Model file for the job. Use its own axes, mm. A direction names the side the tool comes from. Round coordinates to 2 decimals unless told otherwise and drop trailing zeros. Order: outer loops, then holes, each group sorted by start corner. A loop starts at its lowest first (then second) coordinate and runs counter-clockwise, first axis right, second up. Notation, with made-up numbers: (29, 55) -> (60, 55) arc R14 ccw to (60, 76) -> close; hole circle Ø8 at (-14, -20.75). An arc over 180 degrees is marked (long way). Put each result on its own line as item: value. Start each with the question number.
Q1. Cut at A-A, the plane x = 0. List the corners of the cut face in (y, z).
Q2. Probe L1, parallel to X at y = 2.45, z = -11.5; L2, parallel to X at y = 2, z = -11; L3, parallel to X at y = 2.85, z = 12. List the from-to ranges inside material, lowest first.
Q3. Cut at B-B, the plane z = -11.5. List the corners of the cut face in (x, y).
Q4. Flat gauge pins, fed straight in: P1, Ø4, axis at x = 10, z = -11.5, coming from the -Y side; P2, Ø13.5, axis at y = 20, z = 7, coming from the +X side; P3, Ø8, axis at x = -0.5, z = -3.5, coming from the +Y side. Where does each tip first touch, or does it go through?
Q5. Cut at D-D, the plane z = 32. List the corners of the cut face in (x, y).
Q6. Cut at C-C, the plane y = 14.5. List the corners of the cut face in (x, z), and give its area (3 significant figures).
Q7. 3-axis set-ups, long thin cutter, end or side, ignore diameter. For faces 1 (the face through (9.3, 4.1, 29.8)), 2 (the face through (0, 0, 0)), 3 (the face through (7.866, 17.487, 17.458)), 4 (the face through (2.28, 31.85, -43.52)): which of +Z, -Z, +X, -X, +Y, -Y reach the whole face in a straight line?
Q8. Pull direction Z, two halves, no side cores. Call faces 5 (the face through (0, 2.3, 30)), 6 (the face through (0, 7, 45.5)), 7 (the face through (10, 4, -11)): released by +Z, released by -Z, zero draft, split by the parting line, or undercut.
from build123d import *

# Parameters (mm, degrees)
SKETCH_1_W          = 29
SKETCH_1_H          = 29
EXTRUDE_1_DEPTH     = 29
SKETCH_2_R          = 1.7
CUT_EXTRUDE_1_DEPTH = 4
SKETCH_3_R          = 14
EXTRUDE_2_DEPTH     = 12.7
SKETCH_4_R          = 17.5
EXTRUDE_3_DEPTH     = 32.6
SKETCH_6_R          = 19.5
EXTRUDE_4_DEPTH     = 10
CHAMFER_1_SIZE      = 2.5
FILLET_1_R          = 1
SKETCH_7_W          = 22
SKETCH_7_H          = 8.6
EXTRUDE_5_DEPTH     = 31
SKETCH_8_R          = 4.35
EXTRUDE_6_DEPTH     = 6
CHAMFER_2_SIZE      = 3.5


with BuildPart() as part:
    # 草图1 → 凸台-拉伸1 (new body)
    with BuildSketch(Plane(origin=(0, 0, 0), x_dir=(1, 0, 0), z_dir=(0, 1, 0))):
        Rectangle(SKETCH_1_W, SKETCH_1_H)
    extrude(amount=EXTRUDE_1_DEPTH)

    # 草图2 → 切除-拉伸1 (cut)
    with BuildSketch(Plane.XZ):
        with Locations(Location((-10, -11.5, 0), (0, 0, 270))):
            Circle(SKETCH_2_R)
        with Locations(Location((10, -11.5, 0), (0, 0, 270))):
            Circle(SKETCH_2_R)
        with Locations(Location((0, 12, 0), (0, 0, 270))):
            Circle(SKETCH_2_R)
    extrude(amount=-CUT_EXTRUDE_1_DEPTH, mode=Mode.SUBTRACT)

    # 草图3 → 凸台-拉伸2 (add)
    with BuildSketch(Plane(origin=(0, 0, -14.5), x_dir=(-1, 0, 0), z_dir=(0, 0, -1))):
        with Locations((0, 14.5)):
            Circle(SKETCH_3_R)
    extrude(amount=EXTRUDE_2_DEPTH)

    # 草图4 → 凸台-拉伸3 (add)
    with BuildSketch(Plane(origin=(0, 0, -27.2), x_dir=(-1, 0, 0), z_dir=(0, 0, -1))):
        with Locations((0, 14.5)):
            Circle(SKETCH_4_R)
    extrude(amount=EXTRUDE_3_DEPTH)

    # 草图6 → 凸台-拉伸4 (add)
    with BuildSketch(Plane(origin=(0, 0, -59.8), x_dir=(-1, 0, 0), z_dir=(0, 0, -1))):
        with Locations((0, 14.5)):
            Circle(SKETCH_6_R)
    extrude(amount=EXTRUDE_4_DEPTH)

    # 倒角1
    # the kernel refuses this chamfer: 2.5 mm, written as the material it takes off along each edge
    with BuildSketch(Plane(origin=(0, 14.5, -59.8), x_dir=(-1, 0, 0), z_dir=(0, -1, 0))) as chamfer_1_piece_1_section:
        Polygon((19.5, CHAMFER_1_SIZE), (19.5 - CHAMFER_1_SIZE, 0), (19.5, 0), align=None)
    chamfer_1_piece_1 = revolve(axis=Axis((0, 14.5, -59.8), (0, 0, -1)), mode=Mode.PRIVATE)
    chamfer_1_piece_1 = chamfer_1_piece_1 - Plane(origin=(0, 14.5, -61.283957384), x_dir=(-1, 0, 0), z_dir=(0, 0, 1)) * Cylinder(17.5, 78, mode=Mode.PRIVATE)
    add(chamfer_1_piece_1, mode=Mode.SUBTRACT)

    # 圆角1
    fillet_1_edges = [part.edges().sort_by_distance(p)[0] for p in [
        (-14.5, 29, 0),
        (14.5, 29, 0),
        (-14.5, 0, 0),
        (14.5, 0, 0),
    ]]
    fillet(fillet_1_edges, radius=FILLET_1_R)

    # 草图7 → 凸台-拉伸5 (add)
    with BuildSketch(Plane.XY.offset(14.5)):
        with Locations((0, 6.6)):
            Rectangle(SKETCH_7_W, SKETCH_7_H)
    extrude(amount=EXTRUDE_5_DEPTH)

    # 草图8 → 凸台-拉伸6 (add)
    with BuildSketch(Plane.XY.offset(14.5)):
        with Locations(Location((7.3, 21.8, 0), (0, 0, 180))):
            Circle(SKETCH_8_R)
    extrude(amount=EXTRUDE_6_DEPTH)

    # 倒角2
    chamfer_2_edges = [part.edges().sort_by_distance(p)[0] for p in [
        (-11, 10.9, 30),
        (-11, 2.3, 30),
        (11, 2.3, 30),
        (11, 10.9, 30),
    ]]
    chamfer(chamfer_2_edges, length=CHAMFER_2_SIZE)


solid = part.part
Ans:
1. outline: (-5, -69.8) -> (34, -69.8) -> (34, -62.3) -> (32, -60.3) -> (32, -27.2) -> (28.5, -27.2) -> (28.5, -14.5) -> (29, -14.5) -> (29, 14.5) -> (10.9, 14.5) -> (10.9, 45.5) -> (2.3, 45.5) -> (2.3, 14.5) -> (0, 14.5) -> (0, 13.7) -> (4, 13.7) -> (4, 10.3) -> (0, 10.3) -> (0, -14.5) -> (0.5, -14.5) -> (0.5, -27.2) -> (-3, -27.2) -> (-3, -60.3) -> (-5, -62.3) -> close
2. L1: x = -14.5 to -11.7, -8.3 to 8.3, 11.7 to 14.5
2. L2: x = -14.5 to -11.62, -8.38 to 8.38, 11.62 to 14.5
2. L3: x = -14.5 to -1.7, 1.7 to 14.5
3. outline: (-14.5, 1) arc R1 ccw to (-13.5, 0) -> (-11.7, 0) -> (-11.7, 4) -> (-8.3, 4) -> (-8.3, 0) -> (8.3, 0) -> (8.3, 4) -> (11.7, 4) -> (11.7, 0) -> (13.5, 0) arc R1 ccw to (14.5, 1) -> (14.5, 28) arc R1 ccw to (13.5, 29) -> (-13.5, 29) arc R1 ccw to (-14.5, 28) -> close
4. P1: stops at y = 0
4. P2: stops at x = 14.5
4. P3: stops at y = 29
5. outline: (-11, 5.8) -> (-7.5, 2.3) -> (7.5, 2.3) -> (11, 5.8) -> (11, 7.4) -> (7.5, 10.9) -> (-7.5, 10.9) -> (-11, 7.4) -> close
6. outline: (-19.5, -69.8) -> (19.5, -69.8) -> (19.5, -62.3) -> (17.5, -60.3) -> (17.5, -27.2) -> (14, -27.2) -> (14, -14.5) -> (14.5, -14.5) -> (14.5, 14.5) -> (-14.5, 14.5) -> (-14.5, -14.5) -> (-14, -14.5) -> (-14, -27.2) -> (-17.5, -27.2) -> (-17.5, -60.3) -> (-19.5, -62.3) -> close
6. area: 2,720 mm^2
7. face 1: +Z, +X, -Y
7. face 2: +Z, +X, -X, -Y
7. face 3: +Z
7. face 4: none
8. face 5: zero draft
8. face 6: released by +Z
8. face 7: undercut
